Input: part model. Units: mm. Frame: model coordinates. A direction names the side the tool comes from. Give positions to 0.01 mm unless a question says otherwise; leave off trailing zeros. Order: outer loops, then holes, each group sorted by start corner. A loop starts at its lowest first (then second) coordinate and runs counter-clockwise, first axis right, second up. Notation, with made-up numbers: (78, 22) - (112, 22) arc R22 cw to (112, 33) - close; hole circle Ø1 at (56.5, 71). An arc over 180 degrees is marked (long way). Answer in a Markdown table with one row per item. Add a question column.
1. Section query D-D on x = 5. Return loops of the section in (y, z).
2. Mould query, pull axis Z, two halves, no side actions, for faces 4 (the face through (89.614, 1.726, -0.208)), 5 (the face through (94.45, 2, -27)), 6 (the face through (2.75, 2.13, -15.54)), 7 (the face through (93.473, 2.071, -33.223)). Classes: released by +Z, released by -Z, zero draft, split by the parting line, or undercut.
3. Section query A-A on z = -36. Return loops of the section in (x, y), and give its area (3 significant figures).
4. Contact query for flat-ended pins moving along their axis: pin 1 (5 mm diameter, centred on x = 41.5, z = 6, fed in from +Y); pin 2 (0.8 mm diameter, centred on x = 1.5, y = 1, fed in from -Z); pin 3 (0.8 mm diameter, centred on x = 3.5, y = 1, fed in from +Z); pin 4 (1.2 mm diameter, centred on y = 3, z = -40.5, fed in from +X). Output: stop coordinate, or through.
5. Section query C-C on y = 0.8. Count the separate pieces of the cut face and the enclosed holes in it, and give its area (3 significant figures).
6. Section query B-B on x = 66. Return loops of the section in (y, z), and give its area (3 significant figures).
7. Access query for faces 1 (the face through (89.75, 3, -39)), 2 (the face through (1.45, 3, -39)), 3 (the face through (88.4, 1, -29)). Directions: +Z, -Z, +X, -X, +Y, -Y. A direction counts if a zero-diameter tool reaches every point of the face in a straight line with its end or side. Return the directions, or none.
8. Ray query, line 1 (X direction, y = 0.7, z = 0); line 2 (X direction, y = 3, z = 9); line 3 (Z direction, x = 80, y = 2.55). Return the intervals inside material, ascending. Write a range as [from, to].
```python
from build123d import *

# Parameters (mm, degrees)
CROQUIS1_R              = 1.6
SALIENTE_EXTRUIR1_DEPTH = 4.5
SALIENTE_EXTRUIR2_DEPTH = 2.7
CORTAR_EXTRUIR1_DEPTH   = 65.504030882
REDONDEO1_R             = 3
CHAFL_N1_SIZE           = 1
CROQUIS6_W              = 1.15
CROQUIS6_H              = 6.95
CORTAR_EXTRUIR3_DEPTH   = 105.891432104
REDONDEO4_R             = 2
REDONDEO5_R             = 2
CROQUIS7_R              = 1.6
CORTAR_EXTRUIR4_DEPTH   = 105.891432104
CHAFL_N2_SIZE           = 1
CROQUIS8_W              = 75.1
CROQUIS8_H              = 50.1
SALIENTE_EXTRUIR4_DEPTH = 0.8
MOVER_START             = 4.2
MOVER_CARA1_OUTLINE_W   = 75.1
MOVER_CARA1_OUTLINE_H   = 50.1
MOVER_CARA1_DEPTH       = 0.3


# Read off the part's stored shape, not the designer's step: Mover cara1
with BuildPart() as part:
    # Croquis1 → Saliente-Extruir1 (new body)
    with BuildSketch(Plane(origin=(0, 0, 0), x_dir=(1, 0, 0), z_dir=(0, 1, 0))):
        with BuildLine():
            Line((-3.25, 30.9), (-3.25, 0))
            ThreePointArc((-3.25, 0), (-2.298097039, -2.298097039), (0, -3.25))
            Line((0, -3.25), (2.8, -3.25))
            Line((2.8, -3.25), (2.8, 7.7))
            Line((2.8, 7.7), (3.8, 7.7))
            Line((3.8, 7.7), (3.8, 23.2))
            Line((3.8, 23.2), (2.8, 23.2))
            Line((2.8, 23.2), (2.8, 34.15))
            Line((2.8, 34.15), (0, 34.15))
            ThreePointArc((0, 34.15), (-2.298097039, 33.198097039), (-3.25, 30.9))
        make_face()
        with Locations(Location((0, 0, 0), (0, 0, 270))):
            Circle(CROQUIS1_R, mode=Mode.SUBTRACT)
        with Locations(Location((0, 30.9, 0), (0, 0, 270))):
            Circle(CROQUIS1_R, mode=Mode.SUBTRACT)
    extrude(amount=SALIENTE_EXTRUIR1_DEPTH)

    # Croquis2 → Saliente-Extruir2 (add)
    with BuildSketch(Plane(origin=(0, 4.5, 0), x_dir=(1, 0, 0), z_dir=(0, 1, 0))):
        Polygon((45.6, -14.5), (1.45, -14.5), (1.45, 45.4), (45.6, 45.4), (45.6, 42.9), (3.95, 42.9), (3.95, -12), (45.6, -12), align=None)
    extrude(amount=-SALIENTE_EXTRUIR2_DEPTH)

    # Croquis3 → Cortar-Extruir1 (cut, through all)
    with BuildSketch(Plane(origin=(0, 4.5, 0), x_dir=(1, 0, 0), z_dir=(0, 1, 0))):
        with BuildLine():
            Line((-2, 10.7), (-3.25, 10.7))
            Line((-3.25, 10.7), (-3.25, 20.2))
            Line((-3.25, 20.2), (-2, 20.2))
            ThreePointArc((-2, 20.2), (2.75, 15.45), (-2, 10.7))
        make_face()
    extrude(amount=-CORTAR_EXTRUIR1_DEPTH, mode=Mode.SUBTRACT)

    # Simetría1: part across plane


with BuildPart() as part_1:
    add(part.part)
    add(part.part.mirror(Plane(origin=(45.6, -74.412582941, 12), x_dir=(0, 0, 1), z_dir=(1, 0, 0))))

    # Redondeo1
    redondeo1_edges = [part_1.edges().sort_by_distance(p)[0] for p in [
        (94.45, 2.25, -20.2),
        (94.45, 2.25, -10.7),
        (-3.25, 2.25, -20.2),
        (-3.25, 2.25, -10.7),
    ]]
    fillet(redondeo1_edges, radius=REDONDEO1_R)

    # Chaflán1
    chafl_n1_edges = [part_1.edges().sort_by_distance(p)[0] for p in [
        (89.75, 3.15, -45.4),
        (89.75, 3.15, 14.5),
        (1.45, 3.15, 14.5),
        (1.45, 3.15, -45.4),
    ]]
    chamfer(chafl_n1_edges, length=CHAFL_N1_SIZE)

    # Croquis6 → Cortar-Extruir3 (cut, through all)
    with BuildSketch(Plane(origin=(0, 4.5, 0), x_dir=(1, 0, 0), z_dir=(0, 1, 0))):
        with Locations((3.375, 2.975)):
            Rectangle(CROQUIS6_W, CROQUIS6_H)
        with Locations((87.825, 27.925)):
            Rectangle(CROQUIS6_W, CROQUIS6_H)
    extrude(amount=-CORTAR_EXTRUIR3_DEPTH, mode=Mode.SUBTRACT)

    # Redondeo4
    # the kernel refuses this fillet: 2 mm, written as the material it adds along each edge
    with BuildSketch(Plane(origin=(88.4, 4.5, -24.45), x_dir=(0, 0, -1), z_dir=(0, -1, 0)), Plane(origin=(2.8, 4.5, -6.45), x_dir=(0, 0, 1), z_dir=(0, -1, 0))) as redondeo4_piece_1:
        with BuildLine():
            CenterArc((1.810386699, -2), REDONDEO4_R, 90, 64.849336587)
            Line((0, -1.15), (-0.036207734, -1.133))
            ThreePointArc((-0.036207734, -1.133), (-0.04, -0.575), (-0.04, 0))
            Line((-0.04, 0), (0, 0.04))
            Line((0, 0.04), (1.810386699, 0.04))
            Line((1.810386699, 0.04), (1.810386699, 0))
        make_face()
    extrude(amount=2.7)
    with BuildSketch(Plane(origin=(88.4, 4.5, -31.4), x_dir=(-1, 0, 0), z_dir=(0, -1, 0)), Plane(origin=(2.8, 4.5, 0.5), x_dir=(1, 0, 0), z_dir=(0, -1, 0))) as redondeo4_piece_2:
        with BuildLine():
            CenterArc((2, -1.810386699), REDONDEO4_R, 115.150663413, 64.849336587)
            Line((0, -1.810386699), (-0.04, -1.810386699))
            Line((-0.04, -1.810386699), (-0.04, 0))
            Line((-0.04, 0), (0, 0.04))
            ThreePointArc((0, 0.04), (0.575, 0.04), (1.133, 0.036207734))
            Line((1.133, 0.036207734), (1.15, 0))
        make_face()
    extrude(amount=2.7)

    # Redondeo5
    redondeo5_edges = [part_1.edges().sort_by_distance(p)[0] for p in [
        (3.95, 3.15, 0.5),
        (3.95, 3.15, -6.45),
        (87.25, 3.15, -31.4),
        (87.25, 3.15, -24.45),
    ]]
    fillet(redondeo5_edges, radius=REDONDEO5_R)

    # Croquis7 → Cortar-Extruir4 (cut, through all)
    with BuildSketch(Plane.XZ):
        with Locations(Location((0, -30.9, 0), (0, 0, 90))):
            Circle(CROQUIS7_R)
        with Locations(Location((0, 0, 0), (0, 0, 90))):
            Circle(CROQUIS7_R)
        with Locations(Location((91.2, -30.9, 0), (0, 0, 90))):
            Circle(CROQUIS7_R)
        with Locations(Location((91.2, 0, 0), (0, 0, 90))):
            Circle(CROQUIS7_R)
    extrude(amount=-CORTAR_EXTRUIR4_DEPTH, mode=Mode.SUBTRACT)

    # Chaflán2
    chafl_n2_edges = [part_1.edges().sort_by_distance(p)[0] for p in [
        (91.2, 4.5, -32.5),
        (91.2, 4.5, -1.6),
        (0, 4.5, -32.5),
        (0, 4.5, -1.6),
    ]]
    chamfer(chafl_n2_edges, length=CHAFL_N2_SIZE)

    # Croquis8 → Saliente-Extruir4 (add)
    with BuildSketch(Plane(origin=(0, 4.5, 0), x_dir=(1, 0, 0), z_dir=(0, 1, 0))):
        with BuildLine():
            Line((3.95, 42.9), (87.25, 42.9))
            Line((87.25, 42.9), (87.25, 32.396301741))
            ThreePointArc((87.25, 32.396301741), (87.399324448, 31.638014197), (87.825, 30.992957521))
            ThreePointArc((87.825, 30.992957521), (88.250675552, 30.347900845), (88.4, 29.589613301))
            Line((88.4, 29.589613301), (88.4, 26.260386699))
            ThreePointArc((88.4, 26.260386699), (88.250675552, 25.502099155), (87.825, 24.857042479))
            ThreePointArc((87.825, 24.857042479), (87.399324448, 24.211985803), (87.25, 23.453698259))
            Line((87.25, 23.453698259), (87.25, -12))
            Line((87.25, -12), (3.95, -12))
            Line((3.95, -12), (3.95, -1.496301741))
            ThreePointArc((3.95, -1.496301741), (3.800675552, -0.738014197), (3.375, -0.092957521))
            ThreePointArc((3.375, -0.092957521), (2.949324448, 0.552099155), (2.8, 1.310386699))
            Line((2.8, 1.310386699), (2.8, 4.639613301))
            ThreePointArc((2.8, 4.639613301), (2.949324448, 5.397900845), (3.375, 6.042957521))
            ThreePointArc((3.375, 6.042957521), (3.800675552, 6.688014197), (3.95, 7.446301741))
            Line((3.95, 7.446301741), (3.95, 42.9))
        make_face()
        with Locations((48, 15.45)):
            Rectangle(CROQUIS8_W, CROQUIS8_H, mode=Mode.SUBTRACT)
    extrude(amount=-SALIENTE_EXTRUIR4_DEPTH)

    # Mover cara1 outline → Mover cara1 (cut)
    with BuildSketch(Plane(origin=(0, 0, 0), x_dir=(1, 0, 0), z_dir=(0, 1, 0)).offset(MOVER_START)):
        with BuildLine():
            Line((0, -3.25), (1.45, -3.25))
            Line((1.45, -3.25), (1.45, -13.5))
            Line((1.45, -13.5), (2.45, -14.5))
            Line((2.45, -14.5), (88.75, -14.5))
            Line((88.75, -14.5), (89.75, -13.5))
            Line((89.75, -13.5), (89.75, -3.25))
            Line((89.75, -3.25), (91.2, -3.25))
            ThreePointArc((91.2, -3.25), (93.498097039, -2.298097039), (94.45, 0))
            Line((94.45, 0), (94.45, 7.900165565))
            ThreePointArc((94.45, 7.900165565), (93.798644084, 9.766678615), (92.127419355, 10.82268212))
            ThreePointArc((92.127419355, 10.82268212), (88.45, 15.45), (92.127419355, 20.07731788))
            ThreePointArc((92.127419355, 20.07731788), (93.798644084, 21.133321385), (94.45, 22.999834435))
            Line((94.45, 22.999834435), (94.45, 30.9))
            ThreePointArc((94.45, 30.9), (93.498097039, 33.198097039), (91.2, 34.15))
            Line((91.2, 34.15), (89.75, 34.15))
            Line((89.75, 34.15), (89.75, 44.4))
            Line((89.75, 44.4), (88.75, 45.4))
            Line((88.75, 45.4), (2.45, 45.4))
            Line((2.45, 45.4), (1.45, 44.4))
            Line((1.45, 44.4), (1.45, 34.15))
            Line((1.45, 34.15), (0, 34.15))
            ThreePointArc((0, 34.15), (-2.298097039, 33.198097039), (-3.25, 30.9))
            Line((-3.25, 30.9), (-3.25, 22.999834435))
            ThreePointArc((-3.25, 22.999834435), (-2.598644084, 21.133321385), (-0.927419355, 20.07731788))
            ThreePointArc((-0.927419355, 20.07731788), (2.75, 15.45), (-0.927419355, 10.82268212))
            ThreePointArc((-0.927419355, 10.82268212), (-2.598644084, 9.766678615), (-3.25, 7.900165565))
            Line((-3.25, 7.900165565), (-3.25, 0))
            ThreePointArc((-3.25, 0), (-2.298097039, -2.298097039), (0, -3.25))
        make_face()
        with Locations((48, 15.45)):
            Rectangle(MOVER_CARA1_OUTLINE_W, MOVER_CARA1_OUTLINE_H, mode=Mode.SUBTRACT)
    extrude(amount=MOVER_CARA1_DEPTH, mode=Mode.SUBTRACT)


solid = part_1.part
```
Answer:
| question | item | result |
|---|---|---|
| 1 | outline | (1.8, -45.4) - (4.2, -45.4) - (4.2, 14.5) - (1.8, 14.5) - (1.8, 12) - (3.7, 12) - (3.7, -42.9) - (1.8, -42.9) - close |
| 2 | face 4 | undercut |
| 2 | face 5 | zero draft |
| 2 | face 6 | undercut |
| 2 | face 7 | released by -Z |
| 3 | outline | (1.45, 1.8) - (3.95, 1.8) - (3.95, 3.7) - (10.45, 3.7) - (10.45, 4.2) - (1.45, 4.2) - close; (85.55, 3.7) - (87.25, 3.7) - (87.25, 1.8) - (89.75, 1.8) - (89.75, 4.2) - (85.55, 4.2) - close |
| 3 | area | 16.1 mm² |
| 4 | pin 1 | passes through |
| 4 | pin 2 | stops at z = -34.15 |
| 4 | pin 3 | stops at z = -7.7 |
| 4 | pin 4 | stops at x = 89.75 |
| 5 | separate pieces | 2 |
| 5 | enclosed holes | 4 |
| 5 | area | 342 mm² |
| 6 | outline | (1.8, -45.4) - (4.2, -45.4) - (4.2, -40.5) - (3.7, -40.5) - (3.7, -42.9) - (1.8, -42.9) - close; (1.8, 12) - (3.7, 12) - (3.7, 9.6) - (4.2, 9.6) - (4.2, 14.5) - (1.8, 14.5) - close |
| 6 | area | 14.4 mm² |
| 7 | face 1 | -Z, +X, +Y, -Y |
| 7 | face 2 | -Z, -X, +Y, -Y |
| 7 | face 3 | -Y |
| 8 | line 1 | x = [-3.25, -1.6], [1.6, 2.8], [88.4, 89.6], [92.8, 94.45] |
| 8 | line 2 | x = [1.45, 3.95], [87.25, 89.75] |
| 8 | line 3 | z = [-45.4, -42.9], [12, 14.5] |
